Build history of the part. All positions in model axes, mm. A direction names the side the tool comes from. Round coordinates to 2 decimals unless told otherwise and drop trailing zeros. Order: outer loops, then holes, each group sorted by start corner. A loop starts at its lowest first (then second) coordinate and runs counter-clockwise, first axis right, second up. Notation, with made-up numbers: (70.25, -12) -> (83.25, -12) arc R16 cw to (83.25, 4) -> close; hole circle Ø7 at (83, -23.5). An arc over 180 degrees is marked (long way). Answer as a JSON object with one key per item and string values.
from build123d import *

# Parameters (mm, degrees)
SKETCH1_R           = 49.5046
BOSS_EXTRUDE1_DEPTH = 3.175
SKETCH2_R           = 47.6885
BOSS_EXTRUDE2_DEPTH = 3.175
SKETCH3_R           = 6.35
SKETCH3_R_2         = 3.175
CUT_EXTRUDE1_DEPTH  = 71.297463271


with BuildPart() as part:
    # Sketch1 → Boss-Extrude1 (new body)
    with BuildSketch(Plane.XY):
        Circle(SKETCH1_R)
    extrude(amount=BOSS_EXTRUDE1_DEPTH)

    # Sketch2 → Boss-Extrude2 (add)
    with BuildSketch(Plane.XY.offset(3.175)):
        Circle(SKETCH2_R)
    extrude(amount=BOSS_EXTRUDE2_DEPTH)

    # Sketch3 → Cut-Extrude1 (cut, through all)
    with BuildSketch(Plane.XY.offset(6.35)):
        with Locations((-12.7, -31.235352443)):
            Circle(SKETCH3_R)
        with Locations((12.7, -31.235352443)):
            Circle(SKETCH3_R)
        with Locations((-34.925, 0)):
            Circle(SKETCH3_R_2)
        with Locations((34.925, 0)):
            Circle(SKETCH3_R_2)
    extrude(amount=-CUT_EXTRUDE1_DEPTH, mode=Mode.SUBTRACT)


solid = part.part
1) Cut at D-D, the plane z = 2. Give the cut face in (x, y) (3 decimals).
Checked values:
{"outline": "circle Ø99.009 at (0, 0); hole circle Ø6.35 at (-34.925, 0); hole circle Ø12.7 at (-12.7, -31.235); hole circle Ø12.7 at (12.7, -31.235); hole circle Ø6.35 at (34.925, 0)"}
2) Pull direction X, two halves, no side cores. Call faces 1 (the face through (-6.445, 49.083, 1.565)), 2 (the face through (37.953, 0.954, 3.219)), 3 (the face through (-1, 1, 0)): pulls with the +X half, pulls with the -X half, needs draft (parallel to the pull), parting line crosses it, or undercut.
Checked values:
{"face 1": "parting line crosses it", "face 2": "undercut", "face 3": "needs draft"}
3) Flat gauge pins, fed straight in: pin 1 Ø1 at (y, z) = (38.5, 2) entering from -X; pin 2 Ø1.5 at (x, z) = (-1, 5.5) entering from -Y; pin 3 Ø2 at (y, z) = (-34, 2.5) entering from -X. Where does each tip first touch, or does it go through?
Checked values:
{"pin 1": "stops at x = -31.73", "pin 2": "stops at y = -47.69", "pin 3": "stops at x = -36.9"}
4) Probe L1, parallel to Y at x = 17, z = 2.5; L2, parallel to Y at x = -8.5, z = 4.75; L3, parallel to Z at x = 17.5, y = 45.5 (3 decimals). List the from-to ranges inside material, lowest first. Write a range as from..to.
Checked values:
{"L1": "y = -46.49..-35.91, -26.56..46.49", "L2": "y = -46.92..-36, -26.47..46.92", "L3": "z = 0..3.175"}
5) Which spindle directions (+Z, -Z, +X, -X, +Y, -Y) get a long thin tool onto all of the face, cutting with end or side? Do faces 4 (the face through (-13.53, -24.94, 3.22)), 5 (the face through (45.486, 14.324, 4.74)). Say none if no direction does.
Checked values:
{"face 4": "+Z, -Z", "face 5": "+Z"}
6) Cut at A-A, the plane y = 0. Count the separate pieces of the cut face and the enclosed holes in it, plus the area to 3 significant figures.
Checked values:
{"separate pieces": "3", "enclosed holes": "0", "area": "537 mm²"}
